Part model, mm, in its own coordinate system. Coordinates: 2 decimals unless noted, no trailing zeros. Order: outer loops, then holes, each group sorted by start corner. A loop starts at its lowest first (then second) coordinate and runs counter-clockwise, first axis right, second up. Notation, with made-up numbers: M 52,-10.5 L 108,-10.5 A32 cw 108,21.5 Z; hole C 17,69.5 d10. An arc over 180 degrees is marked long. Answer in a Markdown table with one row per item. Add a question column.
from build123d import *

# Parameters (mm, degrees)
BOSS_EXTRUDE1_DEPTH = 22


with BuildPart() as part:
    # Sketch1 → Boss-Extrude1 (new body)
    with BuildSketch(Plane.XY):
        with BuildLine():
            Line((-21.35205925, 11.1154812), (-17.368827213, 20.661456443))
            Line((-17.368827213, 20.661456443), (-21.868827213, 12.867227809))
            ThreePointArc((-21.868827213, 12.867227809), (-21.948667572, 12.73617279), (-22.097868544, 12.700270549))
            Line((-22.097868544, 12.700270549), (-22.196215152, 12.715900014))
            ThreePointArc((-22.196215152, 12.715900014), (-22.326689682, 12.79594909), (-22.362345861, 12.94481176))
            Line((-22.362345861, 12.94481176), (-22.354687101, 12.993003628))
            ThreePointArc((-22.354687101, 12.993003628), (-22.363718798, 13.030380728), (-22.396614586, 13.050292692))
            Line((-22.396614586, 13.050292692), (-22.592962298, 13.079890225))
            ThreePointArc((-22.592962298, 13.079890225), (-22.630105552, 13.070679105), (-22.649856554, 13.037901612))
            Line((-22.649856554, 13.037901612), (-22.832052004, 11.829231305))
            ThreePointArc((-22.832052004, 11.829231305), (-22.822704304, 11.791903872), (-22.789609619, 11.772270774))
            Line((-22.789609619, 11.772270774), (-22.592446198, 11.744397206))
            ThreePointArc((-22.592446198, 11.744397206), (-22.555388987, 11.753948603), (-22.535939439, 11.786905866))
            Line((-22.535939439, 11.786905866), (-22.529535655, 11.832202971))
            ThreePointArc((-22.529535655, 11.832202971), (-22.448384623, 11.96650006), (-22.295290569, 12.00090077))
            Line((-22.295290569, 12.00090077), (-22.264046695, 11.995148315))
            ThreePointArc((-22.264046695, 11.995148315), (-22.113475119, 11.869945968), (-22.141972438, 11.6762056))
            Line((-22.141972438, 11.6762056), (-22.365452219, 11.3868424))
            ThreePointArc((-22.365452219, 11.3868424), (-22.405533487, 11.239109704), (-22.329412432, 11.106305176))
            Line((-22.329412432, 11.106305176), (-21.969472499, 10.828317868))
            ThreePointArc((-21.969472499, 10.828317868), (-21.858721207, 10.786937123), (-21.743952077, 10.81533187))
            Line((-21.743952077, 10.81533187), (-21.441501697, 10.997697404))
            ThreePointArc((-21.441501697, 10.997697404), (-21.385493263, 11.048018041), (-21.35205925, 11.1154812))
        make_face()
    extrude(amount=-BOSS_EXTRUDE1_DEPTH)


solid = part.part
(1) Wall check: line 1 (X direction, y = 19, z = -6.5); line 2 (X direction, y = 18.5, z = -6); line 3 (Y direction, x = -18.1, z = -16.5). Give the ranges that are in metal, low to high.
(2) Slice it at C-C (x = -18.6). List the corners of the cut face in (y, z), and give its area (3 significant figures).
(3) Slice it at B-B (y = 18). List the corners of the cut face in (x, z).
(4) Drop a flat-ended pin along its axis: P1, Ø3, axis at y = 14.5, z = -15.5, coming from the -X side. Give the stop position or say it passes through.
Computed:
| question | item | result |
|---|---|---|
| 1 | line 1 | x = -18.33 to -18.06 |
| 1 | line 2 | x = -18.62 to -18.27 |
| 1 | line 3 | y = 18.91 to 19.4 |
| 2 | outline | M 17.71,-22 L 18.53,-22 L 18.53,0 L 17.71,0 Z |
| 2 | area | 18.0 mm^2 |
| 3 | outline | M -18.91,-22 L -18.48,-22 L -18.48,0 L -18.91,0 Z |
| 4 | P1 | stops at x = -22.66 |
